Verification items for this drawing (mm, ordinates from the low corner). A direction names the side the tool comes from. Round coordinates to 2 decimals unless told otherwise and drop trailing zeros. Order: outer loops, then holes, each group sorted by start corner. A loop starts at its lowest first (then second) coordinate and runs counter-clockwise, first axis right, second up. Notation, with made-up numbers: (16, -32.75) -> (37, -32.75) arc R21 cw to (37, 3.25) -> close; hole circle Ø10 at (70, 35). An arc over 180 degrees is marked (long way). Return JSON: item names as keys, results as strings. Group by question number.
Item 1: Sectioned sample at A-A on y = 12. Record the cut outline in (x, z), plus the area to 3 significant figures.
Item 2: Sectioned sample at C-C on z = 11.25. Record the cut outline in (x, y).
Item 3: Access from +Z, -Z, +X, -X, +Y, -Y to the whole of each face (thin tool, end or side, straight path). Record for the marked faces 1 and 2.
Item 4: Sectioned sample at D-D on y = 2.25. Record the cut outline in (x, z).
Item 5: Sectioned sample at B-B on x = 11. Record the cut outline in (y, z).
Item 6: Draft check along Z on the marked faces 3, 4 and 5. Enter one of: pulls with the +Z half, pulls with the -Z half, needs draft (parallel to the pull), parting line crosses it, or undercut.
Item 7: Depth check by flat-ended pin: pin 1 Ø1.5 at (x, y) = (13.5, 2.5) entering from -Z; pin 2 Ø4.5 at (x, y) = (8.54, 12) entering from -Z; pin 3 Ø12 at (x, z) = (6.5, 15.5) entering from +Y. Enter the tip coordinate at first touch or a pass-through.
Item 8: Scan lines: probe 1 along X at (y, z) = (1, 15); probe 2 along Y at (x, z) = (18, 2.75); probe 3 along Z at (x, y) = (4.5, 17.25). Record each from-to range of solid material in increasing order. Write a range as from..to.
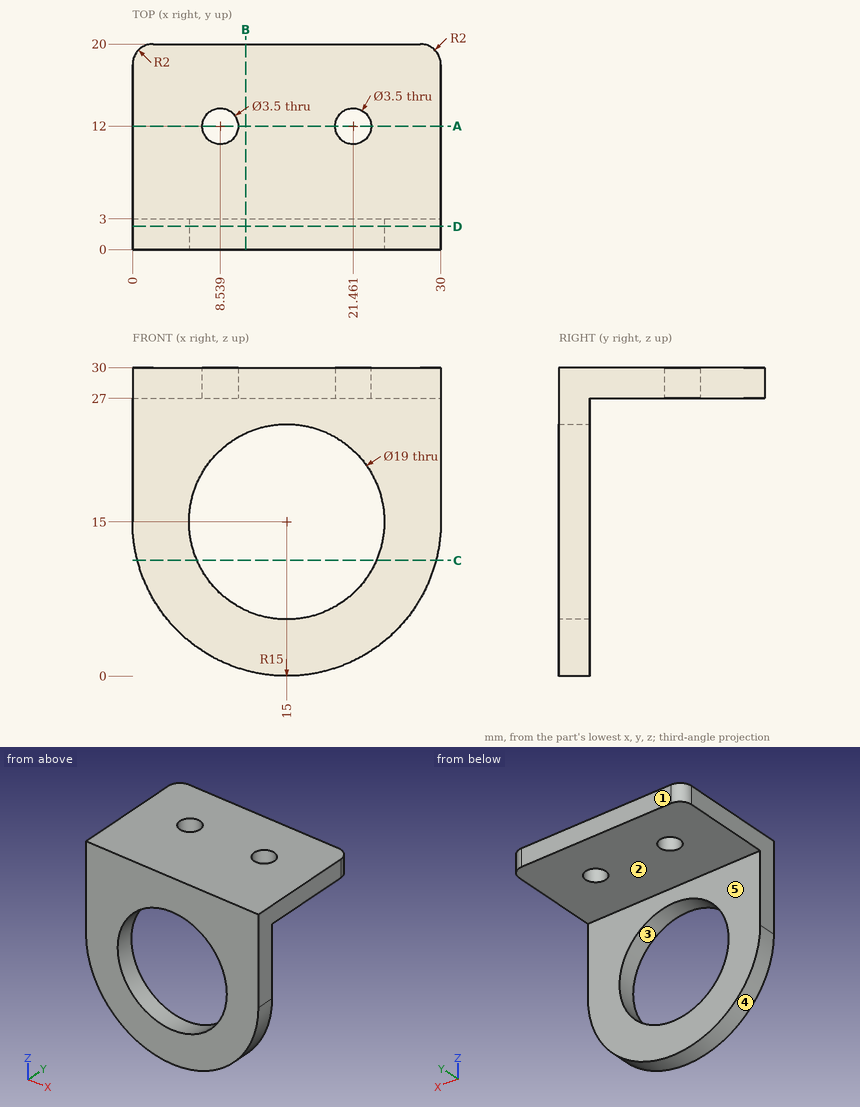
Recorded:
{
 "1": {"outline": "(0, 27) -> (6.79, 27) -> (6.79, 30) -> (0, 30) -> close; (10.29, 27) -> (19.71, 27) -> (19.71, 30) -> (10.29, 30) -> close; (23.21, 27) -> (30, 27) -> (30, 30) -> (23.21, 30) -> close", "area": "69.0 mm²"},
 "2": {"outline": "(0.48, 0) -> (6.27, 0) -> (6.27, 3) -> (0.48, 3) -> close; (23.73, 0) -> (29.52, 0) -> (29.52, 3) -> (23.73, 3) -> close"},
 "3": {"face 1": "+Z, -Z, +X, -X, +Y", "face 2": "-Z, +X, -X, +Y"},
 "4": {"outline": "(0, 15) arc R15 ccw to (30, 15) -> (30, 30) -> (0, 30) -> close; hole circle Ø19 at (15, 15)"},
 "5": {"outline": "(0, 0.54) -> (3, 0.54) -> (3, 6.38) -> (0, 6.38) -> close; (0, 23.62) -> (3, 23.62) -> (3, 27) -> (20, 27) -> (20, 30) -> (0, 30) -> close"},
 "6": {"face 3": "undercut", "face 4": "pulls with the -Z half", "face 5": "needs draft"},
 "7": {"pin 1": "z = 0.02", "pin 2": "z = 27", "pin 3": "y = 3"},
 "8": {"probe 1": "0..5.5, 24.5..30", "probe 2": "0..3", "probe 3": "27..30"}
}
